```python
from build123d import *

# Parameters (mm, degrees)
SKETCH2_R           = 14
BOSS_EXTRUDE1_DEPTH = 2
SKETCH1_W           = 8
SKETCH1_H           = 22.649954628
SKETCH1_W_2         = 6
SKETCH1_H_2         = 18.4
BOSS_EXTRUDE2_DEPTH = 25
SKETCH3_W           = 8
SKETCH3_H           = 22.649954628
BOSS_EXTRUDE3_DEPTH = 5.5
SKETCH4_W           = 6
SKETCH4_H           = 18.4
CUT_EXTRUDE1_DEPTH  = 37.362755671
SKETCH5_W           = 5
SKETCH5_H           = 18.4
CUT_EXTRUDE2_DEPTH  = 40.258756985
SKETCH7_R           = 0.75
CUT_EXTRUDE3_DEPTH  = 44.515565904
BOSS_EXTRUDE4_DEPTH = 30.5
SKETCH9_W           = 3.5
SKETCH9_H           = 7
CUT_EXTRUDE4_DEPTH  = 6


with BuildPart() as part:
    # Sketch2 → Boss-Extrude1 (new body)
    with BuildSketch(Plane.XY):
        Circle(SKETCH2_R)
    extrude(amount=BOSS_EXTRUDE1_DEPTH)

    # Sketch1 → Boss-Extrude2 (add)
    with BuildSketch(Plane.XY.offset(2)):
        Rectangle(SKETCH1_W, SKETCH1_H)
        Rectangle(SKETCH1_W_2, SKETCH1_H_2, mode=Mode.SUBTRACT)
    extrude(amount=BOSS_EXTRUDE2_DEPTH)

    # Sketch3 → Boss-Extrude3 (add)
    with BuildSketch(Plane.XY.offset(27)):
        Rectangle(SKETCH3_W, SKETCH3_H)
    extrude(amount=BOSS_EXTRUDE3_DEPTH)

    # Sketch4 → Cut-Extrude1 (cut, through all)
    with BuildSketch(Plane.XY.offset(2)):
        Rectangle(SKETCH4_W, SKETCH4_H)
    extrude(amount=-CUT_EXTRUDE1_DEPTH, mode=Mode.SUBTRACT)

    # Sketch5 → Cut-Extrude2 (cut, through all)
    with BuildSketch(Plane.ZY.offset(-3)):
        with Locations((24.5, 0)):
            Rectangle(SKETCH5_W, SKETCH5_H)
    extrude(amount=CUT_EXTRUDE2_DEPTH, mode=Mode.SUBTRACT)

    # Sketch7 → Cut-Extrude3 (cut, through all)
    with BuildSketch(Plane(origin=(0, 11.324977314, 0), x_dir=(1, 0, 0), z_dir=(0, 1, 0))):
        with Locations(Location((0, -29.75, 0), (0, 0, 180))):
            Circle(SKETCH7_R)
    extrude(amount=-CUT_EXTRUDE3_DEPTH, mode=Mode.SUBTRACT)

    # Sketch8 → Boss-Extrude4 (add)
    with BuildSketch(Plane.XY.offset(2)):
        with BuildLine():
            Line((4, 11.324977314), (4, -11.324977314))
            Line((4, -11.324977314), (8.23072833, -11.324977314))
            ThreePointArc((8.23072833, -11.324977314), (12.474578081, -6.354911619), (14, 0))
            ThreePointArc((14, 0), (12.474578081, 6.354911619), (8.23072833, 11.324977314))
            Line((8.23072833, 11.324977314), (4, 11.324977314))
        make_face()
    extrude(amount=BOSS_EXTRUDE4_DEPTH)

    # Sketch9 → Cut-Extrude4 (cut)
    with BuildSketch(Plane.XY.offset(32.5)):
        with Locations((5.75, 0)):
            Rectangle(SKETCH9_W, SKETCH9_H)
    extrude(amount=-CUT_EXTRUDE4_DEPTH, mode=Mode.SUBTRACT)


solid = part.part
```
Could you check a few things on this model? Use its own coordinates, in mm. A direction names the side the tool comes from. Give positions to 0.01 mm unless a question says otherwise; leave off trailing zeros. Order: outer loops, then holes, each group sorted by start corner. A loop starts at its lowest first (then second) coordinate and runs counter-clockwise, first axis right, second up.
Q1. If I drill on line 1 along Y through (x, z) = (1.5, 9.5); line 2 along Z through (x, y) = (0, -2.25); line 3 along Y through (x, z) = (-3.25, 18), over which ranges is the centre line in solid material (lowest first)?
Q2. Suppose I cut it at A-A, the plane z = 29.75. Write out the boundary of the cut face in (x, y), and give its area (3 significant figures).
Q3. Suppose I cut it at B-B, the plane x = 0. Write out the boundary of the cut face in (y, z).
Q4. For faces 4 (the flat face through (-3, 0, 11)), 5 (the flat face through (6, -3.5, 30)), 6 (the flat face through (2, -11.325, 17)), which set-ups out of +Z, -Z, +X, -X, +Y, -Y let a thin tool reach every point of the face, with its end or its side?
Q5. I'm going to push flat-ended pins straight in: P1, Ø3.5, axis at x = 0, z = 14, coming from the -Y side (3 decimals); P2, Ø1.8, axis at y = 0, z = 29.5, coming from the -X side; P3, Ø1, axis at x = 5.5, z = 28.5, coming from the +Y side (3 decimals); P4, Ø8, axis at x = -8.5, z = 16, coming from the +Y side. Where does each tip first touch, or does it pass through?
Q6. Suppose I cut it at C-C, the plane y = -5. Write out the boundary of the cut face in (x, z).
Q7. Suppose I cut it at D-D, the plane z = 4. Write out the boundary of the cut face in (x, y), and give its area (3 significant figures).
Q8. We'd pull the mould along X, two halves only. Please class faces 1 (the flat face through (-3.5, -0.1, 22)), 2 (the flat face through (-4, 0, 17)), 3 (the flat face through (4, 0, 30)): +X half, -X half, draft (parallel to the pull), parting line (faces both ways), or undercut.
Solution:
1. line 1: y = -11.32 to -9.2, 9.2 to 11.32
1. line 2: z = 27 to 29, 30.5 to 32.5
1. line 3: y = -11.32 to 11.32
2. outline: (-4, -11.32) - (-0.75, -11.32) - (-0.75, 11.32) - (-4, 11.32) - close; (0.75, -11.32) - (8.23, -11.32) arc R14 ccw to (8.23, 11.32) - (0.75, 11.32) - close; hole (4, -3.5) - (7.5, -3.5) - (7.5, 3.5) - (4, 3.5) - close
2. area: 310 mm2
3. outline: (-14, 0) - (-9.2, 0) - (-9.2, 27) - (9.2, 27) - (9.2, 0) - (14, 0) - (14, 2) - (11.32, 2) - (11.32, 29) - (-11.32, 29) - (-11.32, 2) - (-14, 2) - close; (-11.32, 30.5) - (11.32, 30.5) - (11.32, 32.5) - (-11.32, 32.5) - close
4. face 4: -Z
4. face 5: +Z
4. face 6: +Z, +X, -X, -Y
5. P1: stops at y = -11.325
5. P2: stops at x = -4
5. P3: stops at y = 11.325
5. P4: passes through
6. outline: (-13.08, 0) - (-3, 0) - (-3, 22) - (-4, 22) - (-4, 2) - (-13.08, 2) - close; (-4, 27) - (3, 27) - (3, 0) - (13.08, 0) - (13.08, 32.5) - (-4, 32.5) - close; hole circle Ø1.5 at (0, 29.75)
7. outline: (-4, -11.32) - (8.23, -11.32) arc R14 ccw to (8.23, 11.32) - (-4, 11.32) - close; hole (-3, -9.2) - (3, -9.2) - (3, 9.2) - (-3, 9.2) - close
7. area: 258 mm2
8. face 1: draft
8. face 2: -X half
8. face 3: undercut
